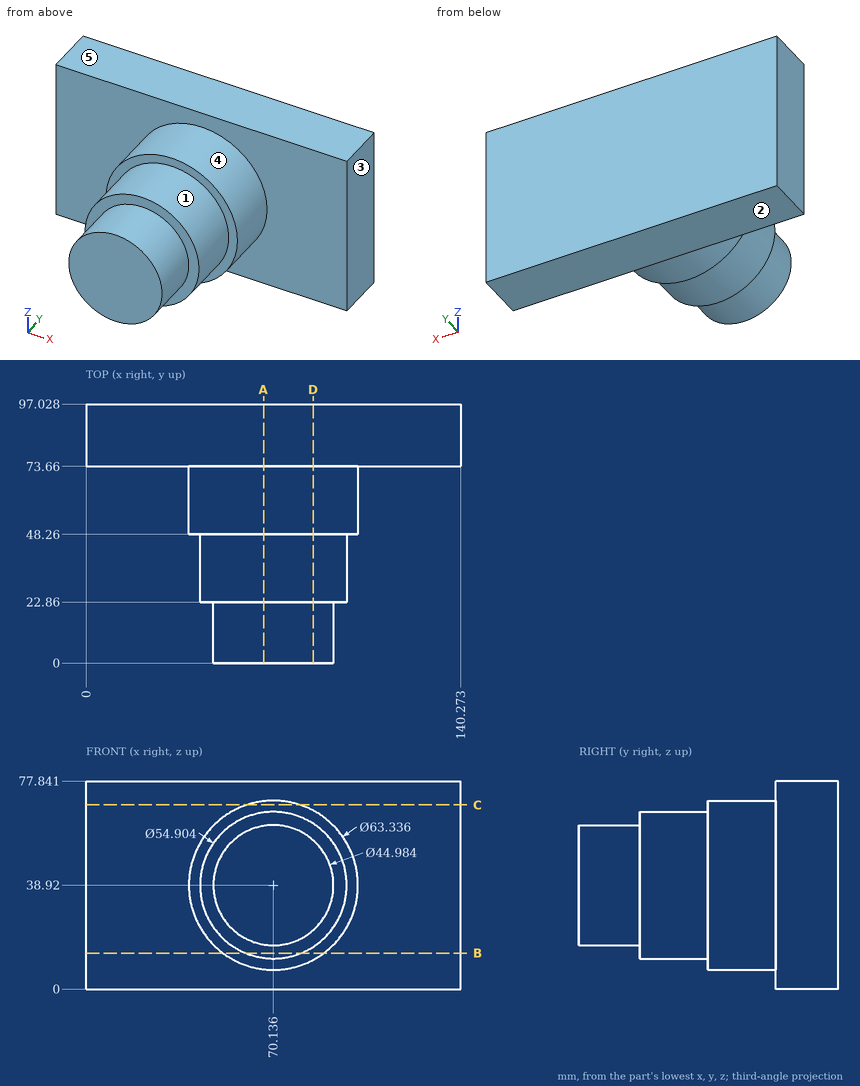
Geometry check sheet. Reference: drawing and pictorial views, mm from the part's lowest x, y, z. A direction names the side the tool comes from. Give positions to 0.01 mm unless a question says otherwise; leave off trailing zeros. Order: outer loops, then holes, each group sorted by start corner. A loop starts at its lowest first (then second) coordinate and runs counter-clockwise, first axis right, second up. Notation, with made-up numbers: (69.5, 52) -> (86.5, 52) arc R17 ccw to (86.5, 78) -> close; hole circle Ø3 at (-21.5, 89). An arc over 180 degrees is marked (long way). Use CSV: the item, a comma, the result in double quotes. Start each with the question number.
1) Mould release check, pull along X, two halves, no side actions. Record for the marked faces 3, 4 and 5: released by +X, released by -X, zero draft, split by the parting line, or undercut.
2) Sectioned sample at C-C, the plane z = 69. Record the boundary of the cut face in (x, y), plus the area to 3 significant figures.
3) Go/stop test with flat-tipped pins: P1, Ø23.5, axis at x = 55, z = 50, coming from the -Y side; P2, Ø1.5, axis at x = 52.5, y = 14, coming from the +Z side; P3, Ø5, axis at x = 70, y = 53, coming from the -Z side; P4, Ø12, axis at y = 23, z = 49.5, coming from the -X side. Record where each tip stops, or that it passes through.
4) Sectioned sample at D-D, the plane x = 85. Record the boundary of the cut face in (y, z), plus the area to 3 significant figures.
5) Material ranges on line 1 (Y direction, x = 44, z = 72.5); line 2 (Y direction, x = 96, z = 40); line 3 (X direction, y = 66.5, z = 19.5), recorded low to high. Write a range as from..to.
6) Sectioned sample at A-A, the plane x = 66.5. Record the boundary of the cut face in (y, z) (1 decimal).
7) Set-up check for the marked faces 1 and 2: record each of +Z, -Z, +X, -X, +Y, -Y from which the full face is reachable in a straight line by a thin tool's end or side.
8) Sectioned sample at B-B, the plane z = 13.5. Record the boundary of the cut face in (x, y), plus the area to 3 significant figures.
Recorded:
1,face 3,"released by +X"
1,face 4,"split by the parting line"
1,face 5,"zero draft"
2,outline,"(0, 73.66) -> (60.23, 73.66) -> (60.23, 48.26) -> (80.04, 48.26) -> (80.04, 73.66) -> (140.27, 73.66) -> (140.27, 97.03) -> (0, 97.03) -> close"
2,area,"3,780 mm2"
3,P1,"y = 0"
3,P2,"z = 53.78"
3,P3,"z = 7.25"
3,P4,"x = 43.07"
4,outline,"(0, 22.04) -> (22.86, 22.04) -> (22.86, 15.84) -> (48.26, 15.84) -> (48.26, 10.96) -> (73.66, 10.96) -> (73.66, 0) -> (97.03, 0) -> (97.03, 77.84) -> (73.66, 77.84) -> (73.66, 66.88) -> (48.26, 66.88) -> (48.26, 62) -> (22.86, 62) -> (22.86, 55.8) -> (0, 55.8) -> close"
4,area,"5,180 mm2"
5,line 1,"73.66..97.03"
5,line 2,"22.86..97.03"
5,line 3,"45.12..95.15"
6,outline,"(0, 16.7) -> (22.9, 16.7) -> (22.9, 11.7) -> (48.3, 11.7) -> (48.3, 7.5) -> (73.7, 7.5) -> (73.7, 0) -> (97, 0) -> (97, 77.8) -> (73.7, 77.8) -> (73.7, 70.4) -> (48.3, 70.4) -> (48.3, 66.1) -> (22.9, 66.1) -> (22.9, 61.1) -> (0, 61.1) -> close"
7,face 1,"-Y"
7,face 2,"-Z, +X, -X, +Y, -Y"
8,outline,"(0, 73.66) -> (51.25, 73.66) -> (51.25, 48.26) -> (59.77, 48.26) -> (59.77, 22.86) -> (80.5, 22.86) -> (80.5, 48.26) -> (89.02, 48.26) -> (89.02, 73.66) -> (140.27, 73.66) -> (140.27, 97.03) -> (0, 97.03) -> close"
8,area,"4,760 mm2"
